Verification items for the finished model (mm, model axes). A direction names the side the tool comes from. Give positions to 0.01 mm unless a question says otherwise; leave off trailing zeros. Write each loop counter-clockwise with the first axis right and the second up, starting at its lowest first coordinate (ties: lowest second). Pieces come first, ordered by that corner, then holes. Notation, with made-up numbers: (-35.5, -25.75) -> (6.5, -25.75) arc R32 cw to (6.5, 13.25) -> close; hole circle Ø2 at (-32.75, -40). An arc over 180 degrees is marked (long way). Write item = value, one per line.
from build123d import *

# Parameters (mm, degrees)
F0_W        = 127
F0_H        = 76.2
F1_DEPTH    = 25.4
F2_W        = 38.1
F2_H        = 76.2
F3_DEPTH    = 25.4
F4_T1_DEPTH = 251.1217558139
F6_DEPTH    = 12.7


# Not quite as in the source:
# - a fillet or chamfer that OpenCascade refuses, or shapes differently, is made with other operations: its cross-section is extruded or revolved along the edge and cut away or added


with BuildPart() as f1:
    # F0 (on Top) → F1 (new body)
    with BuildSketch(Plane.XY):
        with Locations((-4.94965637, -2.3779198527)):
            Rectangle(F0_W, F0_H)
    extrude(amount=F1_DEPTH)

    # F2 (on face) → F3 (join)
    with BuildSketch(Plane.XY.offset(25.4)):
        with Locations((8.6990555257, -2.3779198527)):
            Rectangle(F2_W, F2_H)
    extrude(amount=F3_DEPTH)

    # F4: fillet of radius 36.7926146906 on 1 edges, made by hand

    # F4_s2 → F4_t1 (cut)
    with BuildSketch(Plane.XZ.offset(-123.1829580542)):
        with BuildLine():
            ThreePointArc((27.7490555257, 25.4), (14.3810455558, 43.7803644885), (-7.2352956371, 50.8))
            Line((-7.2352956371, 50.8), (27.7490555257, 50.8))
            Line((27.7490555257, 50.8), (27.7490555257, 25.4))
        make_face()
    extrude(amount=F4_T1_DEPTH, mode=Mode.SUBTRACT)

    # F5 (on face) → F6 (cut)
    with BuildSketch(Plane.XY.offset(25.4)):
        Polygon((-39.4003004222, 23.0220801473), (-60.7068873942, 23.0220801473), (-60.7068873942, -27.7779198527), (-39.4003004222, -27.7779198527), (-17.6245812327, -27.7779198527), (-17.6245812327, 23.0220801473), align=None)
    extrude(amount=-F6_DEPTH, mode=Mode.SUBTRACT)


solid = f1.part
Item 1: Sectioned sample at C-C on y = -15. Record the cut outline in (x, z), then the cut area to 3 significant figures.
Response values:
outline = (-68.45, 0) -> (58.55, 0) -> (58.55, 25.4) -> (27.75, 25.4) arc R36.79 ccw to (-7.24, 50.8) -> (-10.35, 50.8) -> (-10.35, 25.4) -> (-17.62, 25.4) -> (-17.62, 12.7) -> (-60.71, 12.7) -> (-60.71, 25.4) -> (-68.45, 25.4) -> close
area = 3,410 mm^2
Item 2: Set-up check for faces 1 (the flat face through (-39, 23.022, 19)), 2 (the flat face through (-40, 24, 25.4)), 3 (the flat face through (43, -2, 25.4)), 4 (the flat face through (-9, -2, 50.8)), 5 (the flat face through (-68.45, -3, 13)): record each of +Z, -Z, +X, -X, +Y, -Y from which the full face is reachable in a straight line by a thin tool's end or side.
Response values:
face_1 = +Z
face_2 = +Z, -X, +Y, -Y
face_3 = +Z, +X, +Y, -Y
face_4 = +Z, +X, -X, +Y, -Y
face_5 = +Z, -Z, -X, +Y, -Y
Item 3: Sectioned sample at D-D on z = 36.5. Record the cut outline in (x, y).
Response values:
outline = (-10.35, -40.48) -> (21.88, -40.48) -> (21.88, 35.72) -> (-10.35, 35.72) -> close
Item 4: Sectioned sample at B-B on x = -21.5. Record the cut outline in (y, z).
Response values:
outline = (-40.48, 0) -> (35.72, 0) -> (35.72, 25.4) -> (23.02, 25.4) -> (23.02, 12.7) -> (-27.78, 12.7) -> (-27.78, 25.4) -> (-40.48, 25.4) -> close
Item 5: Go/stop test with flat-tipped pins: P1, Ø7.5, axis at y = 9, z = 33, coming from the -X side; P2, Ø17.5, axis at x = -53, y = -16.5, coming from the +Z side; P3, Ø21.5, axis at x = -46, y = -4.5, coming from the +Z side. Record where each tip stops, or that it passes through.
Response values:
P1 = -10.35
P2 = 25.4
P3 = 12.7
Item 6: Material ranges on line 1 (X direction, y = 11, z = 15); line 2 (Z direction, x = -38, y = -14.5); line 3 (Z direction, x = 33.5, y = 31), recorded low to high.
Response values:
line_1 = -68.45 to -60.71, -17.62 to 58.55
line_2 = 0 to 12.7
line_3 = 0 to 25.4
Item 7: Sectioned sample at A-A on y = 28. Record the cut outline in (x, z), then the cut area to 3 significant figures.
Response values:
outline = (-68.45, 0) -> (58.55, 0) -> (58.55, 25.4) -> (27.75, 25.4) arc R36.79 ccw to (-7.24, 50.8) -> (-10.35, 50.8) -> (-10.35, 25.4) -> (-68.45, 25.4) -> close
area = 3,960 mm^2
Item 8: Mould release check, pull along Y, two halves, no side actions. Record for faces 6 (the flat face through (-6, 35.722, 19)), 7 (the flat face through (-39, -2, 12.7)), 8 (the flat face through (58.55, -3, 13)): +Y half, -Y half, draft (parallel to the pull), parting line (faces both ways), or undercut.
Response values:
face_6 = +Y half
face_7 = undercut
face_8 = draft
